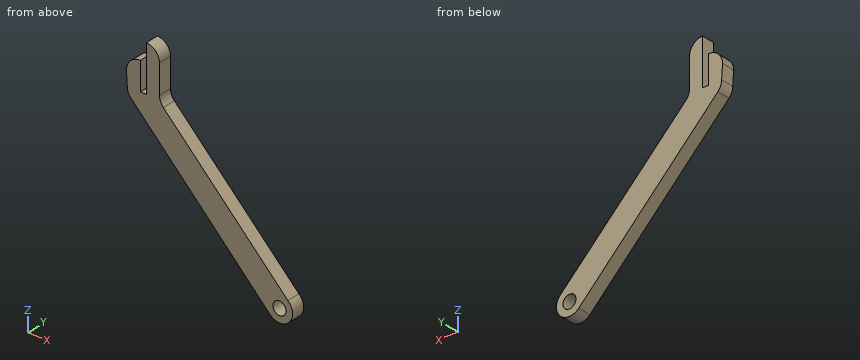
```python
from build123d import *

# Parameters (mm, degrees)
SALIENTE_EXTRUIR1_DEPTH = 10
CROQUIS2_R              = 5
CORTAR_EXTRUIR1_DEPTH   = 11


with BuildPart() as part:
    # Croquis1 → Saliente-Extruir1 (new body)
    with BuildSketch(Plane(origin=(0, 0, 0), x_dir=(1, 0, 0), z_dir=(0, 1, 0))):
        with BuildLine():
            Line((-4.53910409, 0), (0, 0))
            Line((0, 0), (0, -35))
            ThreePointArc((0, -35), (7.071067812, -32.071067812), (10, -25))
            Line((10, -25), (10, -3.173501178))
            ThreePointArc((10, -3.173501178), (10.766393259, 0.665835552), (12.948101308, 3.916683924))
            Line((12.948101308, 3.916683924), (107.92484737, 98.380547972))
            ThreePointArc((107.92484737, 98.380547972), (108.912854015, 112.807521211), (94.455845276, 113.13708499))
            Line((94.455845276, 113.13708499), (-11.610171902, 7.071067812))
            ThreePointArc((-11.610171902, 7.071067812), (-13.777899415, 3.826834324), (-14.53910409, 0))
            Line((-14.53910409, 0), (-15.191410871, -10.652306781))
            ThreePointArc((-15.191410871, -10.652306781), (-12.07142245, -18.18462514), (-4.53910409, -21.304613561))
            Line((-4.53910409, -21.304613561), (-4.53910409, 0))
        make_face()
    extrude(amount=SALIENTE_EXTRUIR1_DEPTH)

    # Croquis2 → Cortar-Extruir1 (cut, through all)
    with BuildSketch(Plane(origin=(0, 10, 0), x_dir=(1, 0, 0), z_dir=(0, 1, 0))):
        with Locations((101.526913088, 106.066017178)):
            Circle(CROQUIS2_R)
    extrude(amount=-CORTAR_EXTRUIR1_DEPTH, mode=Mode.SUBTRACT)


solid = part.part
```
Check sheet for the modelled part. Datum: model origin and axes. Units: mm. Round coordinates to 2 decimals unless told otherwise and drop trailing zeros. Order: outer loops, then holes, each group sorted by start corner. A loop starts at its lowest first (then second) coordinate and runs counter-clockwise, first axis right, second up.
1) Section check A-A (y = 6). Record the boundary of the cut face in (x, z).
2) Section check D-D (z = -10). Record the boundary of the cut face in (x, y), and give its area (3 significant figures).
3) Scan lines: line 1 (Z direction, x = 103, y = 6.25); line 2 (X direction, y = 3.75, z = 14.5); line 3 (X direction, y = 5, z = -88.5). Record each from-to range of solid material in increasing order.
4) Section check C-C (x = 2). Record the boundary of the cut face in (y, z), and give its area (3 significant figures).
5) Go/stop test with flat-tipped pins: pin 1 Ø5 at (y, z) = (6, 12.5) entering from +X; pin 2 Ø1 at (y, z) = (2, -90.5) entering from -X; pin 3 Ø6 at (x, y) = (63, 7.5) entering from -Z. Record where each tip stops, or that it passes through.
6) Section check B-B (z = 9). Record the boundary of the cut face in (x, y).
Result:
1. outline: (-15.19, 10.65) - (-14.54, 0) arc R10 ccw to (-11.61, -7.07) - (94.46, -113.14) arc R10 ccw (long way) to (107.92, -98.38) - (12.95, -3.92) arc R10 cw to (10, 3.17) - (10, 25) arc R10 ccw to (0, 35) - (0, 0) - (-4.54, 0) - (-4.54, 21.3) arc R10.65 ccw to start; hole circle Ø10 at (101.53, -106.07)
2. outline: (-8.68, 0) - (19.06, 0) - (19.06, 10) - (-8.68, 10) - close
2. area: 277 mm2
3. line 1: z = -115.96 to -110.84, -101.29 to -93.48
3. line 2: x = -14.47 to -4.54, 0 to 10
3. line 3: x = 69.82 to 97.99
4. outline: (0, -20.68) - (10, -20.68) - (10, 34.8) - (0, 34.8) - close
4. area: 555 mm2
5. pin 1: stops at x = 10
5. pin 2: stops at x = 71.32
5. pin 3: stops at z = -84.68
6. outline: (-15.09, 0) - (-4.54, 0) - (-4.54, 10) - (-15.09, 10) - close; (0, 0) - (10, 0) - (10, 10) - (0, 10) - close
